The figure shows three views and two pictorial views of one solid part (mm, origin at its lowest corner). Answer the questions. Coordinates: 2 decimals unless noted, no trailing zeros. Order: outer loops, then holes, each group sorted by start corner. A loop starts at its lowest first (then second) coordinate and runs counter-clockwise, first axis right, second up. Notation, with made-up numbers: (8.5, 65) -> (54.5, 65) arc R33 cw to (54.5, 93) -> close; hole circle Ø9 at (47, 68). An arc over 180 degrees is marked (long way). Use one line per item in the form item = value.
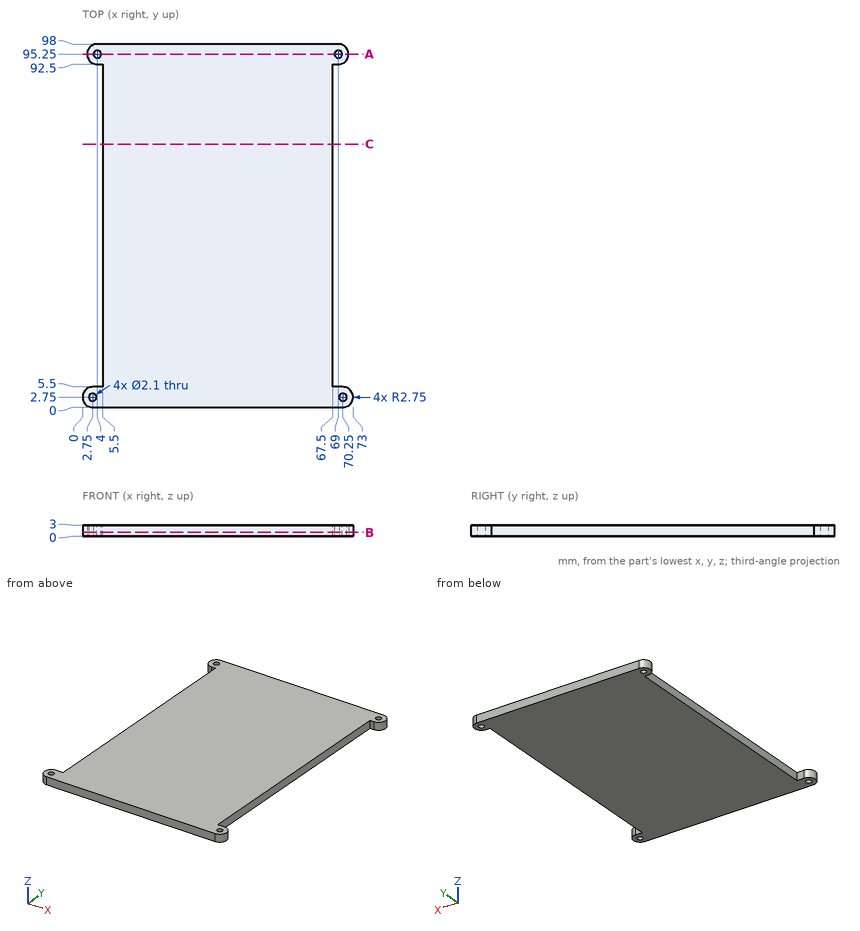
(1) Straight lines are drawn through the part: line 1 along X through (y, z) = (95.25, 2.25); line 2 along Y through (x, z) = (4, 1.8); line 3 along Y through (x, z) = (70.25, 0.85). For each, find the intervals that lie inside material, in ascending order.
Data:
line_1 = 1.25 to 2.95, 5.05 to 67.95, 70.05 to 71.75
line_2 = 0 to 5.5, 92.5 to 94.2, 96.3 to 98
line_3 = 0 to 1.7, 3.8 to 5.5, 92.8 to 97.7
(2) Section B-B on z = 1.1 is taken. Write down the section's boundary in (x, y), plus the area to 3 significant figures.
Data:
outline = (2.75, 0) -> (70.25, 0) arc R2.75 ccw to (70.25, 5.5) -> (67.5, 5.5) -> (67.5, 92.5) -> (69, 92.5) arc R2.75 ccw to (69, 98) -> (4, 98) arc R2.75 ccw to (4, 92.5) -> (5.5, 92.5) -> (5.5, 5.5) -> (2.75, 5.5) arc R2.75 ccw to start; hole circle Ø2.1 at (2.75, 2.75); hole circle Ø2.1 at (4, 95.25); hole circle Ø2.1 at (69, 95.25); hole circle Ø2.1 at (70.25, 2.75)
area = 6,160 mm²
(3) Section C-C on y = 71 is taken. Write down the section's boundary in (x, z).
Data:
outline = (5.5, 0) -> (67.5, 0) -> (67.5, 3) -> (5.5, 3) -> close
(4) Section A-A on y = 95.25 is taken. Write down the section's boundary in (x, z), plus the area to 3 significant figures.
Data:
outline = (1.25, 0) -> (2.95, 0) -> (2.95, 3) -> (1.25, 3) -> close; (5.05, 0) -> (67.95, 0) -> (67.95, 3) -> (5.05, 3) -> close; (70.05, 0) -> (71.75, 0) -> (71.75, 3) -> (70.05, 3) -> close
area = 199 mm²
